Model file for the job. Use its own axes, mm. A direction names the side the tool comes from. Give positions to 0.01 mm unless a question says otherwise; leave off trailing zeros. Loops run counter-clockwise (first coordinate to the right, second up) from the corner with the lowest first, then second, coordinate; pieces in that order, holes last. Notation, with made-up numbers: (-27, 43.25) -> (17, 43.25) arc R19 cw to (17, 60.25) -> close; hole circle Ø5 at (41, 89.5). An arc over 180 degrees is marked (long way). Use CSV: the item, a comma, the result in double quotes. Start each with the question number.
(1) Cut at A-A on x = 17.5. Write the cut outline in (y, z).
(2) Cut at C-C on x = 9.5. Write the cut outline in (y, z), then the cut area to 3 significant figures.
(3) Drill centre lines: probe 1 along Y at (x, z) = (-35, 22); probe 2 along Z at (x, y) = (19, 12.5); probe 3 along Z at (x, y) = (17.5, -31.35). Where is each one in solid material? Low to high.
(4) Cut at D-D on y = -12. Write the cut outline in (x, z), then the cut area to 3 significant figures.
(5) Pull direction X, two halves, no side cores. Call faces 1 (the cylindrical face through (14.914, 31.201, 21.842)), 2 (the flat face through (25.5, -0.2, -0.3)), 3 (the flat face through (-16.765, 31.201, 7.175)), 4 (the flat face through (-4, 31, 33.215)): pulls with the +X half, pulls with the -X half, needs draft (parallel to the pull), parting line crosses it, or undercut.
(6) 3-axis set-ups, long thin cutter, end or side, ignore diameter. For faces 5 (the flat face through (1, -30.215, 16)), 6 (the flat face through (1, 32.215, 16)): which of +Z, -Z, +X, -X, +Y, -Y reach the whole face in a straight line?
(7) Flat gauge pins, fed straight in: pin 1 (7.5 mm diameter, centred on x = 17.5, z = 25.21, fed in from -Y); pin 2 (13.5 mm diameter, centred on x = 18, y = 9, fed in from +Z); pin 3 (1 mm diameter, centred on y = -5, z = -0.5, fed in from -X). Where does each tip first touch, or does it go through?
(8) Cut at B-B on z = 17.5. Write the cut outline in (x, y), then the cut area to 3 significant figures.
from build123d import *

# Parameters (mm, degrees)
SKETCH1_W                  = 75
SKETCH1_H                  = 130
BASE_FLANGE1_DEPTH         = 2
SKETCHED_START             = -37.5
SKETCHED_BEND1_DEPTH       = 75
SKETCHED_BEND1_2_OUTLINE_W = 2
SKETCHED_BEND1_2_OUTLINE_H = 33.214601837
SKETCHED_BEND1_2_DEPTH     = 75
CUT_EXTRUDE1_START         = -64.429203673
CUT_EXTRUDE1_DEPTH         = 64.429203673
CUT_EXTRUDE2_DEPTH         = 82.61238914
CUT_EXTRUDE2_DEPTH_BACK    = 82.61238914
SKETCH9_R                  = 4
CUT_EXTRUDE3_DEPTH         = 82.61238914
CUT_EXTRUDE3_DEPTH_BACK    = 82.61238914
SKETCH10_R                 = 4.25
SKETCH10_W                 = 12
SKETCH10_H                 = 100
FILLET7_R                  = 5


# Read off the part's stored shape, not the designer's step: Sketched Bend1, Cut-Extrude1
# Sheet-metal steps are written as plain solids
with BuildPart() as part:
    # Sketch1 → Base-Flange1 (new body)
    with BuildSketch(Plane.XY):
        Rectangle(SKETCH1_W, SKETCH1_H)
    extrude(amount=-BASE_FLANGE1_DEPTH)

    # Sketched Bend1 outline → Sketched Bend1 (cut)
    with BuildSketch(Plane.YZ.offset(SKETCHED_START)):
        with BuildLine():
            Line((65, 0), (32.214601837, 0))
            ThreePointArc((32.214601837, 0), (31.628815399, -1.414213562), (30.214601837, -2))
            Line((30.214601837, -2), (65, -2))
            Line((65, -2), (65, 0))
        make_face()
        with BuildLine():
            Line((-65, -2), (-30.214601837, -2))
            ThreePointArc((-30.214601837, -2), (-31.628815399, -1.414213562), (-32.214601837, 0))
            Line((-32.214601837, 0), (-65, 0))
            Line((-65, 0), (-65, -2))
        make_face()
    extrude(amount=SKETCHED_BEND1_DEPTH, mode=Mode.SUBTRACT)

    # Sketched Bend1 2 outline → Sketched Bend1 2 (add)
    with BuildSketch(Plane.YZ.offset(SKETCHED_START)):
        with Locations((31.214601837, 16.607300919)):
            Rectangle(SKETCHED_BEND1_2_OUTLINE_W, SKETCHED_BEND1_2_OUTLINE_H)
        with Locations((-31.214601837, 16.607300919)):
            Rectangle(SKETCHED_BEND1_2_OUTLINE_W, SKETCHED_BEND1_2_OUTLINE_H)
    extrude(amount=SKETCHED_BEND1_2_DEPTH)

    # Cut-Extrude1 outline → Cut-Extrude1 (cut)
    with BuildSketch(Plane(origin=(0, 32.214601837, 0), x_dir=(1, 0, 0), z_dir=(0, 1, 0)).offset(CUT_EXTRUDE1_START)):
        with BuildLine():
            Line((-37.5, -33.214601837), (-27.5, -33.214601837))
            ThreePointArc((-27.5, -33.214601837), (-34.571067812, -30.285669649), (-37.5, -23.214601837))
            Line((-37.5, -23.214601837), (-37.5, -33.214601837))
        make_face()
        with BuildLine():
            ThreePointArc((-37.5, -23.214601837), (-35.933914458, -17.841605753), (-31.726182617, -14.151523966))
            Line((-31.726182617, -14.151523966), (-1.378141536, 0))
            Line((-1.378141536, 0), (-1.378141536, 2))
            Line((-1.378141536, 2), (-37.5, 2))
            Line((-37.5, 2), (-37.5, -23.214601837))
        make_face()
    extrude(amount=CUT_EXTRUDE1_DEPTH, mode=Mode.SUBTRACT)

    # Sketch9 → Cut-Extrude2 (cut, two sides: drawn at the far end of the back side and taken through both)
    with BuildSketch(Plane(origin=(0, 32.214601837, 0), x_dir=(1, 0, 0), z_dir=(0, 1, 0)).offset(-CUT_EXTRUDE2_DEPTH_BACK)):
        with Locations(Location((-27.5, -23.214601837, 0), (0, 0, 270))):
            Circle(SKETCH9_R)
    extrude(amount=CUT_EXTRUDE2_DEPTH + CUT_EXTRUDE2_DEPTH_BACK, mode=Mode.SUBTRACT)

    # Sketch10 → Cut-Extrude3 (cut, two sides: drawn at the far end of the back side and taken through both)
    with BuildSketch(Plane(origin=(0, 32.214601837, 0), x_dir=(1, 0, 0), z_dir=(0, 1, 0)).offset(-CUT_EXTRUDE3_DEPTH_BACK)):
        with Locations(Location((17.5, -25.214601837, 0), (0, 0, 270))):
            Circle(SKETCH10_R)
        with Locations((31.5, 16.785398163)):
            Rectangle(SKETCH10_W, SKETCH10_H)
    extrude(amount=CUT_EXTRUDE3_DEPTH + CUT_EXTRUDE3_DEPTH_BACK, mode=Mode.SUBTRACT)

    # Fillet7
    fillet7_edges = [part.edges().sort_by_distance(p)[0] for p in [
        (25.5, 31.214601837, 33.214601837),
        (25.5, -31.214601837, 33.214601837),
    ]]
    fillet(fillet7_edges, radius=FILLET7_R)


solid = part.part
Check result:
1,outline,"(-32.21, 0) arc R2 ccw to (-30.21, -2) -> (30.21, -2) arc R2 ccw to (32.21, 0) -> (32.21, 20.96) -> (30.21, 20.96) -> (30.21, 0) -> (-30.21, 0) -> (-30.21, 20.96) -> (-32.21, 20.96) -> close; (-32.21, 29.46) -> (-30.21, 29.46) -> (-30.21, 33.21) -> (-32.21, 33.21) -> close; (30.21, 29.46) -> (32.21, 29.46) -> (32.21, 33.21) -> (30.21, 33.21) -> close"
2,outline,"(-32.21, 0) arc R2 ccw to (-30.21, -2) -> (30.21, -2) arc R2 ccw to (32.21, 0) -> (32.21, 33.21) -> (30.21, 33.21) -> (30.21, 0) -> (-30.21, 0) -> (-30.21, 33.21) -> (-32.21, 33.21) -> close"
2,area,"260 mm²"
3,probe 1,"-32.21 to -30.21, 30.21 to 32.21"
3,probe 2,"-2 to 0"
3,probe 3,"-1.65 to 20.96, 29.46 to 33.21"
4,outline,"(-1.38, -2) -> (25.5, -2) -> (25.5, 0) -> (-1.38, 0) -> close"
4,area,"53.8 mm²"
5,face 1,"undercut"
5,face 2,"pulls with the +X half"
5,face 3,"pulls with the -X half"
5,face 4,"needs draft"
6,face 5,"+Z, +X, -X"
6,face 6,"+Z, -Z, +X, -X, +Y"
7,pin 1,"through"
7,pin 2,"z = 0"
7,pin 3,"x = -1.38"
8,outline,"(-35.71, -32.21) -> (25.5, -32.21) -> (25.5, -30.21) -> (-35.71, -30.21) -> close; (-35.71, 30.21) -> (25.5, 30.21) -> (25.5, 32.21) -> (-35.71, 32.21) -> close"
8,area,"245 mm²"
